Here's how the part is built. I have some questions about the finished solid (model axes, mm). A direction names the side the tool comes from. Coordinates: 2 decimals unless noted, no trailing zeros. Order: outer loops, then holes, each group sorted by start corner. A loop starts at its lowest first (then second) coordinate and runs counter-clockwise, first axis right, second up. Notation, with made-up numbers: M 2.25,-29 L 14.25,-29 A19 cw 14.25,8 Z; hole C 12,77 d3. An arc over 180 degrees is marked long. One line per question, with ' | ' between items. Start each with the question number.
```python
from build123d import *

# Parameters (mm, degrees)
SKETCH1_W           = 64
SKETCH1_H           = 36
BOSS_EXTRUDE1_DEPTH = 15
FILLET1_R           = 2.5
SKETCH2_RX          = 14.501940206
SKETCH2_RY          = 9.5
BOSS_EXTRUDE2_DEPTH = 1
SKETCH3_R           = 3.563696192
BOSS_EXTRUDE3_DEPTH = 1


with BuildPart() as part:
    # Sketch1 → Boss-Extrude1 (new body)
    with BuildSketch(Plane.XY):
        with Locations((2.310469314, -0.093862816)):
            Rectangle(SKETCH1_W, SKETCH1_H)
    extrude(amount=BOSS_EXTRUDE1_DEPTH)

    # Fillet1
    fillet1_edges = [part.edges().sort_by_distance(p)[0] for p in [
        (-29.689530686, 17.906137184, 7.5),
        (34.310469314, 17.906137184, 7.5),
        (34.310469314, -18.093862816, 7.5),
        (-29.689530686, -18.093862816, 7.5),
    ]]
    fillet(fillet1_edges, radius=FILLET1_R)

    # Sketch2 → Boss-Extrude2 (add)
    with BuildSketch(Plane.XY.offset(15)):
        with Locations(Location((-4.689530686, 0.237212403), (0, 0, 0.937245327))):
            Ellipse(SKETCH2_RX, SKETCH2_RY)
    extrude(amount=BOSS_EXTRUDE2_DEPTH)

    # Sketch3 → Boss-Extrude3 (add)
    with BuildSketch(Plane(origin=(34.310469314, 0, 0), x_dir=(0, 0, -1), z_dir=(1, 0, 0))):
        with Locations((-9.325073978, 0)):
            Circle(SKETCH3_R)
    extrude(amount=BOSS_EXTRUDE3_DEPTH)


solid = part.part
```
1. Imagine slicing it at A-A (z = 7.5). List the corners of the cut face in (x, y) for me, then the cut area to 3 significant figures.
2. Will these pins go through, and if not, where does the flat tip stop? pin 1 (3 mm diameter, centred on x = 8.5, y = -11.5, fed in from -Z); pin 2 (1 mm diameter, centred on x = -20, y = 11, fed in from +Z).
3. Which directions (+Z, -Z, +X, -X, +Y, -Y) give clear straight access to the entire face, cutting with the end or side of a thin tool? Please do faces 1 (the face through (-5, 0, 16)), 2 (the face through (9, 4, 15)), 3 (the face through (34.803, 1.07, 5.926)).
4. Imagine slicing it at C-C (x = 16). List the corners of the cut face in (y, z) for me.
5. I need wall thicknesses on line 1 (Z direction, x = -16, y = -6); line 2 (X direction, y = -3, z = 6.5); line 3 (X direction, y = 1.5, z = 15.25). Which ranges of each line are inside material? Lowest first, please.
6. Imagine slicing it at B-B (y = 14). List the corners of the cut face in (x, z) for me.
Entries:
1) outline: M -29.69,-15.59 A2.5 ccw -27.19,-18.09 L 31.81,-18.09 A2.5 ccw 34.31,-15.59 L 34.31,-3.06 L 35.31,-3.06 L 35.31,3.06 L 34.31,3.06 L 34.31,15.41 A2.5 ccw 31.81,17.91 L -27.19,17.91 A2.5 ccw -29.69,15.41 Z | area: 2,300 mm²
2) pin 1: z = 0 | pin 2: z = 15
3) face 1: +Z, +X, -X, +Y, -Y | face 2: +Z | face 3: +X
4) outline: M -18.09,0 L 17.91,0 L 17.91,15 L -18.09,15 Z
5) line 1: 0 to 15 | line 2: -29.69 to 34.31 | line 3: -19.03 to 9.71
6) outline: M -29.69,0 L 34.31,0 L 34.31,15 L -29.69,15 Z
